Input: part model. Units: mm. Frame: model coordinates. Face numbers are marked on the shaded views. A direction names the side the tool comes from. Coordinates: 2 decimals unless noted, no trailing zeros. Write each loop counter-clockwise with the first axis right and the second up, starting at its lowest first coordinate (ties: lowest second). Pieces come first, ordered by that corner, then holes. Notation, with made-up numbers: (43.5, 50.25) - (47.5, 50.25) arc R25 ccw to (47.5, 65.25) - close; hole circle Ø1 at (-21.5, 43.5). An arc over 180 degrees is marked (long way). Use a Markdown table: item, result. Add a question column.
Q1. Mould query, pull axis X, two halves, no side actions, for the marked faces 1, 2 and 3. Classes: released by +X, released by -X, zero draft, split by the parting line, or undercut.
Q2. Section query C-C (y = 40). Return the cut outline in (x, z).
Q3. Pin query (flat end, axial travel): P1, Ø2, axis at x = 16, y = 52.5, coming from the -Z side; P2, Ø1, axis at y = 58, z = 43, coming from the +X side; P3, Ø6, axis at x = 9, y = 49, coming from the +Z side; P4, Ø9, axis at x = 38.1, z = -14.21, coming from the +Y side. Return the tip coordinate at first contact, or that it passes through.
Q4. Set-up query: the marked faces 4 and 5. Return all of +Z, -Z, +X, -X, +Y, -Y with unobstructed straight access to the full face (end or side cutting, diameter ignored); none if empty.
Q5. Material intervals for probe 1 along Y at (x, z) = (20, -2.5); probe 2 along Z at (x, y) = (19.5, 22.5); probe 3 along Z at (x, y) = (14, 12.5), sorted ascending. Write a range as from..to.
Q6. Section query D-D (z = 88). Return the cut outline in (x, y), then the cut area to 3 significant figures.
Q7. Section query B-B (x = 8.5). Return the cut outline in (y, z), then the cut area to 3 significant figures.
Q8. Section query A-A (x = 44). Return the cut outline in (y, z), then the cut area to 3 significant figures.
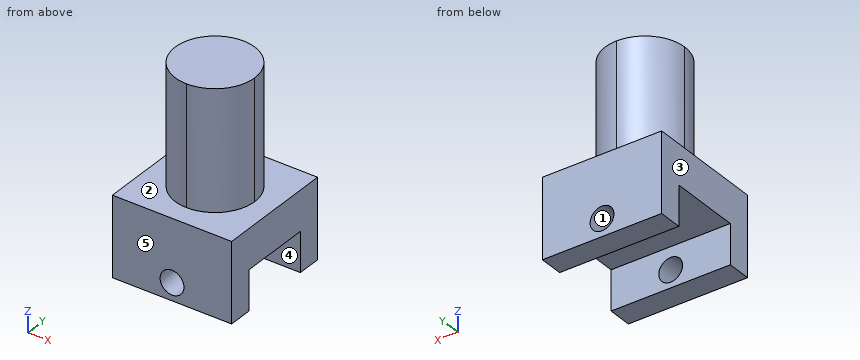
from build123d import *

# Parameters (mm, degrees)
SKETCH5_W           = 76.2
SKETCH5_H           = 76.2
BOSS_EXTRUDE3_DEPTH = 25.4
BOSS_EXTRUDE4_DEPTH = 76.2
SKETCH7_W           = 38.1
SKETCH7_H           = 15.221971119
SKETCH7_H_2         = 15.332492997
BOSS_EXTRUDE5_DEPTH = 25.4
SKETCH8_R           = 7.62
CUT_EXTRUDE1_DEPTH  = 149.106178129


with BuildPart() as part:
    # Sketch5 → Boss-Extrude3 (new body)
    with BuildSketch(Plane.XY):
        with Locations((38.1, 38.1)):
            Rectangle(SKETCH5_W, SKETCH5_H)
    extrude(amount=BOSS_EXTRUDE3_DEPTH)

    # Sketch6 → Boss-Extrude4 (add)
    with BuildSketch(Plane.XY.offset(25.4)):
        with BuildLine():
            ThreePointArc((63.5, 38.1), (56.060512242, 56.060512242), (38.1, 63.5))
            Line((38.1, 63.5), (38.1, 38.1))
            Line((38.1, 38.1), (63.5, 38.1))
        make_face()
        with BuildLine():
            Line((38.1, 38.1), (38.1, 63.5))
            ThreePointArc((38.1, 63.5), (20.139487758, 56.060512242), (12.7, 38.1))
            Line((12.7, 38.1), (38.1, 38.1))
        make_face()
        with BuildLine():
            Line((63.5, 38.1), (38.1, 38.1))
            Line((38.1, 38.1), (38.1, 12.7))
            ThreePointArc((38.1, 12.7), (56.060512242, 20.139487758), (63.5, 38.1))
        make_face()
        with BuildLine():
            Line((38.1, 12.7), (38.1, 38.1))
            Line((38.1, 38.1), (12.7, 38.1))
            ThreePointArc((12.7, 38.1), (20.139487758, 20.139487758), (38.1, 12.7))
        make_face()
    extrude(amount=BOSS_EXTRUDE4_DEPTH)

    # Sketch7 → Boss-Extrude5 (add)
    with BuildSketch(Plane(origin=(0, 0, 0), x_dir=(-1, 0, 0), z_dir=(0, 0, -1))):
        with Locations((-57.15, 68.589014441)):
            Rectangle(SKETCH7_W, SKETCH7_H)
        with Locations((-19.05, 68.589014441)):
            Rectangle(SKETCH7_W, SKETCH7_H)
        with Locations((-57.15, 7.666246499)):
            Rectangle(SKETCH7_W, SKETCH7_H_2)
        with Locations((-19.05, 7.666246499)):
            Rectangle(SKETCH7_W, SKETCH7_H_2)
    extrude(amount=BOSS_EXTRUDE5_DEPTH)

    # Sketch8 → Cut-Extrude1 (cut, through all)
    with BuildSketch(Plane.XZ):
        with Locations(Location((38.1, -14.21368923, 0), (0, 0, 270))):
            Circle(SKETCH8_R)
    extrude(amount=-CUT_EXTRUDE1_DEPTH, mode=Mode.SUBTRACT)


solid = part.part
Values follow:
| question | item | result |
|---|---|---|
| 1 | face 1 | undercut |
| 1 | face 2 | zero draft |
| 1 | face 3 | released by -X |
| 2 | outline | (0, 0) - (76.2, 0) - (76.2, 25.4) - (63.43, 25.4) - (63.43, 101.6) - (12.77, 101.6) - (12.77, 25.4) - (0, 25.4) - close |
| 3 | P1 | z = 0 |
| 3 | P2 | x = 54.5 |
| 3 | P3 | z = 25.4 |
| 3 | P4 | through |
| 4 | face 4 | -Z, +X, -X |
| 4 | face 5 | +Z, -Z, +X, -X, -Y |
| 5 | probe 1 | 0..15.33, 60.98..76.2 |
| 5 | probe 2 | 0..101.6 |
| 5 | probe 3 | -25.4..25.4 |
| 6 | outline | circle Ø50.8 at (38.1, 38.1) |
| 6 | area | 2,030 mm2 |
| 7 | outline | (0, -25.4) - (15.33, -25.4) - (15.33, 0) - (60.98, 0) - (60.98, -25.4) - (76.2, -25.4) - (76.2, 25.4) - (0, 25.4) - close |
| 7 | area | 2,710 mm2 |
| 8 | outline | (0, -25.4) - (15.33, -25.4) - (15.33, -19.04) - (0, -19.04) - close; (0, -9.39) - (15.33, -9.39) - (15.33, 0) - (60.98, 0) - (60.98, -9.39) - (76.2, -9.39) - (76.2, 25.4) - (62.81, 25.4) - (62.81, 101.6) - (13.39, 101.6) - (13.39, 25.4) - (0, 25.4) - close; (60.98, -25.4) - (76.2, -25.4) - (76.2, -19.04) - (60.98, -19.04) - close |
| 8 | area | 6,180 mm2 |
